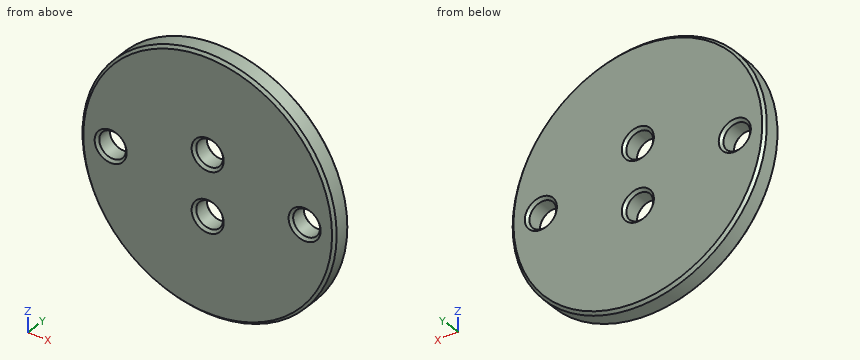
```python
from build123d import *

# Parameters (mm, degrees)
SKETCH1_R           = 19
SKETCH1_R_2         = 2
BOSS_EXTRUDE1_DEPTH = 3
CHAMFER1_SIZE       = 0.4


with BuildPart() as part:
    # Sketch1 → Boss-Extrude1 (new body)
    with BuildSketch(Plane(origin=(0, 0, 0), x_dir=(1, 0, 0), z_dir=(0, 1, 0))):
        Circle(SKETCH1_R)
        with Locations((-14.5, 0)):
            Circle(SKETCH1_R_2, mode=Mode.SUBTRACT)
        with Locations((14.5, 0)):
            Circle(SKETCH1_R_2, mode=Mode.SUBTRACT)
        with Locations((0, 4.5)):
            Circle(SKETCH1_R_2, mode=Mode.SUBTRACT)
        with Locations((0, -4.5)):
            Circle(SKETCH1_R_2, mode=Mode.SUBTRACT)
    extrude(amount=BOSS_EXTRUDE1_DEPTH)

    # Chamfer1
    chamfer1_edges = [part.edges().sort_by_distance(p)[0] for p in [
        (-2, 0, -4.5),
        (-2, 3, -4.5),
        (-2, 0, 4.5),
        (-2, 3, 4.5),
        (-19, 0, 0),
        (-19, 3, 0),
        (-16.5, 0, 0),
        (-16.5, 3, 0),
        (12.5, 0, 0),
        (12.5, 3, 0),
    ]]
    chamfer(chamfer1_edges, length=CHAMFER1_SIZE)


solid = part.part
```
Part model, mm, in its own coordinate system. Coordinates: 2 decimals unless noted, no trailing zeros. Order: outer loops, then holes, each group sorted by start corner. A loop starts at its lowest first (then second) coordinate and runs counter-clockwise, first axis right, second up. Notation, with made-up numbers: (88, 81.5) - (134, 81.5) arc R15 ccw to (134, 94.5) - close; hole circle Ø3 at (14, -4). An arc over 180 degrees is marked (long way). Return JSON: item names as keys, results as strings. Group by question number.
Item 1: Cut at A-A (x = 0). List the corners of the cut face in (y, z).
Item 2: Cut at B-B (z = 0). List the corners of the cut face in (x, y).
Item 3: Drill centre lines: probe 1 along Z at (x, y) = (0, 1.8); probe 2 along X at (y, z) = (1.8, 0); probe 3 along X at (y, z) = (2.8, 1). Where is each one in solid material? Low to high. Write a range as from..to.
Item 4: Cut at C-C (y = 1.15). List the corners of the cut face in (x, z).
Item 5: Pin check, flat tips, straight feed: pin 1 (4.5 mm diameter, centred on x = -14.5, z = 0, fed in from -Y); pin 2 (1.5 mm diameter, centred on y = 1.5, z = 7.5, fed in from -X). Stop position of each tip, or through.
Check values:
{
 "1": {"outline": "(0, -18.6) - (0.4, -19) - (2.6, -19) - (3, -18.6) - (3, -6.9) - (2.6, -6.5) - (0.4, -6.5) - (0, -6.9) - close; (0, -2.1) - (0.4, -2.5) - (2.6, -2.5) - (3, -2.1) - (3, 2.1) - (2.6, 2.5) - (0.4, 2.5) - (0, 2.1) - close; (0, 6.9) - (0.4, 6.5) - (2.6, 6.5) - (3, 6.9) - (3, 18.6) - (2.6, 19) - (0.4, 19) - (0, 18.6) - close"},
 "2": {"outline": "(-19, 0.4) - (-18.6, 0) - (-16.9, 0) - (-16.5, 0.4) - (-16.5, 2.6) - (-16.9, 3) - (-18.6, 3) - (-19, 2.6) - close; (-12.5, 0.4) - (-12.1, 0) - (12.1, 0) - (12.5, 0.4) - (12.5, 2.6) - (12.1, 3) - (-12.1, 3) - (-12.5, 2.6) - close; (16.5, 0.4) - (16.9, 0) - (18.6, 0) - (19, 0.4) - (19, 2.6) - (18.6, 3) - (16.9, 3) - (16.5, 2.6) - close"},
 "3": {"probe 1": "z = -19..-6.5, -2.5..2.5, 6.5..19", "probe 2": "x = -19..-16.5, -12.5..12.5, 16.5..19", "probe 3": "x = -18.77..-16.46, -12.54..12.54, 16.46..18.77"},
 "4": {"outline": "circle Ø38 at (0, 0); hole circle Ø4 at (-14.5, 0); hole circle Ø4 at (0, -4.5); hole circle Ø4 at (0, 4.5); hole circle Ø4 at (14.5, 0)"},
 "5": {"pin 1": "stops at y = 0.15", "pin 2": "stops at x = -17.76"}
}
